```python
from build123d import *

# Parameters (mm, degrees)
EXTRUDE_1_DEPTH     = 78
SKETCH_2_W          = 76.862745098
SKETCH_2_H          = 79.911669522
CUT_EXTRUDE_1_DEPTH = 35
FILLET_1_R          = 1
SKETCH_3_R          = 4.3
CUT_EXTRUDE_2_DEPTH = 35
SKETCH_4_R          = 4.3
CUT_EXTRUDE_3_DEPTH = 35


with BuildPart() as part:
    # 草图1 → 凸台-拉伸1 (new body)
    with BuildSketch(Plane.XY):
        Polygon((0, 0), (-78, 0), (-78, 10), (-70, 10), (-10, 70), (-10, 78), (0, 78), align=None)
    extrude(amount=EXTRUDE_1_DEPTH)

    # 草图2 → 切除-拉伸1 (cut, symmetric)
    with BuildSketch(Plane.XY.offset(39)):
        with Locations((-45.431372549, 46.955834761)):
            Rectangle(SKETCH_2_W, SKETCH_2_H)
    extrude(amount=CUT_EXTRUDE_1_DEPTH, both=True, mode=Mode.SUBTRACT)

    # 圆角1
    fillet_1_edges = [part.edges().sort_by_distance(p)[0] for p in [
        (-78, 10, 76),
        (-10, 78, 76),
        (-78, 10, 2),
        (-10, 78, 2),
    ]]
    fillet(fillet_1_edges, radius=FILLET_1_R)

    # 草图3 → 切除-拉伸2 (cut, symmetric)
    with BuildSketch(Plane(origin=(0, 0, 0), x_dir=(0, 0, -1), z_dir=(1, 0, 0))):
        with Locations(Location((-19, 64, 0), (0, 0, 90))):
            Circle(SKETCH_3_R)
        with Locations(Location((-59, 64, 0), (0, 0, 90))):
            Circle(SKETCH_3_R)
        with BuildLine():
            Line((-14.7, 36.4), (-14.7, 23.9))
            ThreePointArc((-14.7, 23.9), (-19, 19.6), (-23.3, 23.9))
            Line((-23.3, 23.9), (-23.3, 36.4))
            ThreePointArc((-23.3, 36.4), (-19, 40.7), (-14.7, 36.4))
        make_face()
        with BuildLine():
            Line((-54.7, 36.4), (-54.7, 23.9))
            ThreePointArc((-54.7, 23.9), (-59, 19.6), (-63.3, 23.9))
            Line((-63.3, 23.9), (-63.3, 36.4))
            ThreePointArc((-63.3, 36.4), (-59, 40.7), (-54.7, 36.4))
        make_face()
    extrude(amount=CUT_EXTRUDE_2_DEPTH, both=True, mode=Mode.SUBTRACT)

    # 草图4 → 切除-拉伸3 (cut, symmetric)
    with BuildSketch(Plane.XZ):
        with Locations(Location((-64, 59, 0), (0, 0, 270))):
            Circle(SKETCH_4_R)
        with Locations(Location((-64, 19, 0), (0, 0, 270))):
            Circle(SKETCH_4_R)
        with BuildLine():
            Line((-36.4, 63.3), (-23.9, 63.3))
            ThreePointArc((-23.9, 63.3), (-19.6, 59), (-23.9, 54.7))
            Line((-23.9, 54.7), (-36.4, 54.7))
            ThreePointArc((-36.4, 54.7), (-40.7, 59), (-36.4, 63.3))
        make_face()
        with BuildLine():
            Line((-36.4, 23.3), (-23.9, 23.3))
            ThreePointArc((-23.9, 23.3), (-19.6, 19), (-23.9, 14.7))
            Line((-23.9, 14.7), (-36.4, 14.7))
            ThreePointArc((-36.4, 14.7), (-40.7, 19), (-36.4, 23.3))
        make_face()
    extrude(amount=CUT_EXTRUDE_3_DEPTH, both=True, mode=Mode.SUBTRACT)


solid = part.part
```
Work out the finished part from the listing and answer in its coordinate system (mm). A direction names the side the tool comes from. Give positions to 0.01 mm unless a question says otherwise; leave off trailing zeros. Write each loop counter-clockwise with the first axis right and the second up, starting at its lowest first coordinate (ties: lowest second). Pieces come first, ordered by that corner, then holes.
(1) Straight lines are drawn through the part: line 1 (Z direction, x = -4, y = 64); line 2 (X direction, y = 1, z = 59); line 3 (Z direction, x = -8, y = 10). For each, find the intervals that lie inside material, in ascending order.
Final values:
line 1: z = 0 to 14.7, 23.3 to 54.7, 63.3 to 78
line 2: x = -78 to -68.3, -59.7 to -40.7, -19.6 to 0
line 3: z = 0 to 4, 74 to 78
(2) The part is cut by section C-C on y = 34. Write down the section's boundary in (x, z).
Final values:
outline: (-46, 0) - (0, 0) - (0, 14.7) - (-7, 14.7) - (-7, 4) - (-46, 4) - close; (-46, 74) - (-7, 74) - (-7, 63.3) - (0, 63.3) - (0, 78) - (-46, 78) - close; (-7, 23.3) - (0, 23.3) - (0, 54.7) - (-7, 54.7) - close
(3) Which of the six approach directions +Z, -Z, +X, -X, +Y, -Y give full straight-line access (tool end or side, diameter ignored) to faces 1 (the flat face through (-27, 27, 74)), 2 (the flat face through (-74, 10, 2)), 3 (the cylindrical face through (-40.7, 3.5, 18.9))?
Final values:
face 1: -X, +Y
face 2: +Z, -Z, -X, +Y
face 3: +Y, -Y
(4) The part is cut by section D-D on y = 52. Write down the section's boundary in (x, z).
Final values:
outline: (-28, 0) - (0, 0) - (0, 78) - (-28, 78) - (-28, 74) - (-7, 74) - (-7, 4) - (-28, 4) - close
(5) The part is cut by section B-B on z = 19. Write down the section's boundary in (x, y), plus the area to 3 significant figures.
Final values:
outline: (-78, 0) - (-68.3, 0) - (-68.3, 7) - (-78, 7) - close; (-59.7, 0) - (-40.7, 0) - (-40.7, 7) - (-59.7, 7) - close; (-19.6, 0) - (0, 0) - (0, 19.6) - (-7, 19.6) - (-7, 7) - (-19.6, 7) - close; (-7, 40.7) - (0, 40.7) - (0, 59.7) - (-7, 59.7) - close; (-7, 68.3) - (0, 68.3) - (0, 78) - (-7, 78) - close
area: 627 mm2
(6) The mould has two halves that part along Y. Classify faces 4 (the cylindrical face through (-3.5, 68.1, 60.3)), 5 (the flat face through (-43, 7, 39)), 6 (the flat face through (0, 40, 38)), 7 (the cylindrical face through (-3.5, 40.7, 19.1)): pulls with the +Y half, pulls with the -Y half, needs draft (parallel to the pull), parting line crosses it, or undercut.
Final values:
face 4: undercut
face 5: pulls with the +Y half
face 6: needs draft
face 7: undercut
(7) Flat-ended cylindrical pins translate along their axes: pin 1 Ø3 at (y, z) = (74, 2.5) entering from -X; pin 2 Ø4 at (x, z) = (-47.5, 16) entering from +Y. Find the tip coordinate at first contact, or state that the pin passes through.
Final values:
pin 1: stops at x = -10
pin 2: stops at y = 7
(8) The part is cut by section A-A on x = -64. Write down the section's boundary in (y, z).
Final values:
outline: (0, 0) - (16, 0) - (16, 4) - (7, 4) - (7, 14.7) - (0, 14.7) - close; (0, 23.3) - (7, 23.3) - (7, 54.7) - (0, 54.7) - close; (0, 63.3) - (7, 63.3) - (7, 74) - (16, 74) - (16, 78) - (0, 78) - close
